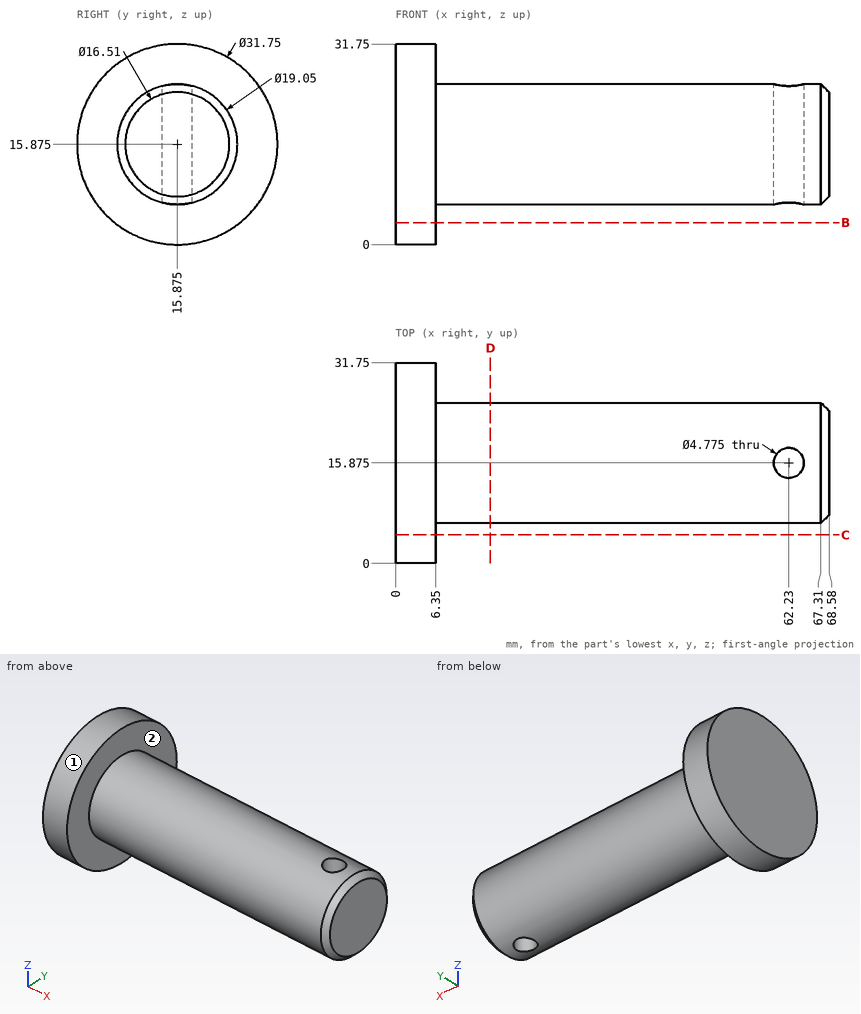
Here's the drawing with two shaded views (mm, measured from the low corner). I have some questions. A direction names the side the tool comes from. Round coordinates to 2 decimals unless told otherwise and drop trailing zeros. Loops run counter-clockwise (first coordinate to the right, second up) from the corner with the lowest first, then second, coordinate; pieces in that order, holes last.
1. Suppose I cut it at C-C, the plane y = 4.5. Please give me the cut outline in (x, z), and give its area (3 significant figures).
Answers:
outline: (0, 4.8) - (6.35, 4.8) - (6.35, 26.95) - (0, 26.95) - close
area: 141 mm2
2. If I drill on probe 1 along Y at (x, z) = (62, 16); probe 2 along X at (y, z) = (6.5, 10.5); probe 3 along Y at (x, z) = (62.23, 20), over which ranges is the centre line in solid material (lowest first)?
Answers:
probe 1: y = 6.35 to 13.5, 18.25 to 25.4
probe 2: x = 0 to 6.35
probe 3: y = 7.29 to 13.49, 18.26 to 24.46
3. Will these pins go through, and if not, where does the flat tip stop? pin 1 (12 mm diameter, centred on x = 52, z = 16, fed in from +Y); pin 2 (1.5 mm diameter, centred on x = 40, y = 27, fed in from +Z); pin 3 (4 mm diameter, centred on x = 28.5, z = 20, fed in from +Y); pin 4 (3 mm diameter, centred on y = 8.5, z = 6.5, fed in from +X).
Answers:
pin 1: stops at y = 25.4
pin 2: passes through
pin 3: stops at y = 25.16
pin 4: stops at x = 6.35
4. Suppose I cut it at D-D, the plane x = 15. Please give me the cut outline in (y, z) (3 decimals), and give its area (3 significant figures).
Answers:
outline: circle Ø19.05 at (15.875, 15.875)
area: 285 mm2
5. Suppose I cut it at B-B, the plane z = 3.5. Please give me the cut outline in (x, y).
Answers:
outline: (0, 5.93) - (6.35, 5.93) - (6.35, 25.82) - (0, 25.82) - close
6. For the marked faces 1 and 2, which set-ups out of +Z, -Z, +X, -X, +Y, -Y let a thin tool reach every point of the face, with its end or its side?
Answers:
face 1: +X, -X
face 2: +X
